For this review, take the finished solid that the model builds, in its own axes (mm). A direction names the side the tool comes from. Give positions to 0.01 mm unless a question says otherwise; leave off trailing zeros. Loops run counter-clockwise (first coordinate to the right, second up) from the corner with the lowest first, then second, coordinate; pieces in that order, holes last. Notation, with made-up numbers: (-8.5, 49.5) -> (31.5, 49.5) arc R16 ccw to (31.5, 55.5) -> close; hole circle Ø4 at (-16.5, 55). An arc over 180 degrees is marked (long way). One line per question, with ' | ' between items. Start each with the question number.
(1) Draft analysis for pull direction X (two halves, no side actions). For faces 1 (the flat face through (-20.3, 2, 0)), 2 (the cylindrical face through (20.72, -20.49, 24.65)), 3 (the cylindrical face through (-17.15, 16.99, 24.65)), state which applies: +X half, -X half, draft (parallel to the pull), parting line (faces both ways), or undercut.
(2) Consider section B-B (y = 375). Write out the cut boundary in (x, z), and give its area (3 significant figures).
(3) Consider section A-A (x = 0). Write out the cut boundary in (y, z), and give its area (3 significant figures).
(4) Insertion check: P1, Ø5, axis at x = 14, z = 31.5, coming from the +Y side; P2, Ø16, axis at x = -4, z = 30.5, coming from the +Y side; P3, Ø5, axis at x = 14.5, y = 231, coming from the +Z side. Each pin has a flat end and moves straight along its axis. Give the tip position at first contact, or say it passes through.
(5) Tool access review of faces 4 (the flat face through (-20.3, 2, 50)), 5 (the flat face through (0, -25, 25)), 6 (the cylindrical face through (-16.99, -17.15, 24.65)): name each direction out of +Z, -Z, +X, -X, +Y, -Y from which nothing blocks a thin tool from reaching the whole face with its end or side.
(6) Consider section C-C (z = 64.5). Write out the cut boundary in (x, y), and give its area (3 significant figures).
(7) Consider section D-D (y = 296). Write out the cut boundary in (x, z), and give its area (3 significant figures).
(8) Wall thickness on probe 1 along Y at (x, z) = (0, 14); probe 2 along Y at (x, z) = (2, 34); probe 3 along Z at (x, y) = (0, 319): over which ranges is each line inside the solid? List them lowest first.
from build123d import *

# Parameters (mm, degrees)
EXTRUDE_1_DEPTH     = 50
SKETCH_2_W          = 40
SKETCH_2_H          = 40
EXTRUDE_2_DEPTH     = 600
FILLET_1_RADIUS     = 20
FILLET_1_LENGTH     = 40
SKETCH_5_R          = 7.5
EXTRUDE_4_DEPTH     = 30
SKETCH_6_R          = 15
CUT_EXTRUDE_1_DEPTH = 631.892225344


with BuildPart() as part:
    # 草图1 → 凸台-拉伸1 (new body)
    with BuildSketch(Plane.XY):
        with BuildLine():
            Line((-10, 25), (10, 25))
            ThreePointArc((10, 25), (20.606601718, 20.606601718), (25, 10))
            Line((25, 10), (25, -10))
            ThreePointArc((25, -10), (20.606601718, -20.606601718), (10, -25))
            Line((10, -25), (-10, -25))
            ThreePointArc((-10, -25), (-20.606601718, -20.606601718), (-25, -10))
            Line((-25, -10), (-25, 10))
            ThreePointArc((-25, 10), (-20.606601718, 20.606601718), (-10, 25))
        make_face()
        with BuildLine():
            Line((-10, 20), (10, 20))
            ThreePointArc((10, 20), (17.071067812, 17.071067812), (20, 10))
            Line((20, 10), (20, -10))
            ThreePointArc((20, -10), (17.071067812, -17.071067812), (10, -20))
            Line((10, -20), (-10, -20))
            ThreePointArc((-10, -20), (-17.071067812, -17.071067812), (-20, -10))
            Line((-20, -10), (-20, 10))
            ThreePointArc((-20, 10), (-17.071067812, 17.071067812), (-10, 20))
        make_face(mode=Mode.SUBTRACT)
    extrude(amount=EXTRUDE_1_DEPTH)

    # 草图2 → 凸台-拉伸2 (add)
    with BuildSketch(Plane(origin=(0, 25, 0), x_dir=(1, 0, 0), z_dir=(0, 1, 0))):
        with Locations((0, -25)):
            Rectangle(SKETCH_2_W, SKETCH_2_H)
    extrude(amount=EXTRUDE_2_DEPTH)

    # 圆角1: full round fillet: the end face becomes a half cylinder, R = half its width
    fillet_1_face = Plane((0, 625, 25), x_dir=(0, 0, -1), z_dir=(0, 1, 0))  # on the end face: x along it, z out of the body
    fillet_1_slab = fillet_1_face.offset(-FILLET_1_RADIUS / 2) * Box(FILLET_1_LENGTH, 2 * FILLET_1_RADIUS, FILLET_1_RADIUS, mode=Mode.PRIVATE)  # the body's end, R deep
    fillet_1_round = Plane((0, 605, 25), x_dir=(0, 1, 0), z_dir=(0, 0, -1)) * Cylinder(FILLET_1_RADIUS, FILLET_1_LENGTH, mode=Mode.PRIVATE)  # its axis R under the face
    add(fillet_1_slab - fillet_1_round, mode=Mode.SUBTRACT)

    # 草图5 → 凸台-拉伸4 (add)
    with BuildSketch(Plane.XY.offset(45)):
        with Locations(Location((0, 605, 0), (0, 0, 180))):
            Circle(SKETCH_5_R)
    extrude_4 = extrude(amount=EXTRUDE_4_DEPTH)

    # 镜向2: 凸台-拉伸4 across plane
    add(extrude_4.mirror(Plane.XY.offset(25)))

    # 草图6 → 切除-拉伸1 (cut, through all)
    with BuildSketch(Plane(origin=(25, 0, 45), x_dir=(1, 0, 0), z_dir=(0, 0, 1))):
        with Locations((-25, 375)):
            Circle(SKETCH_6_R)
    extrude(amount=-CUT_EXTRUDE_1_DEPTH, mode=Mode.SUBTRACT)


solid = part.part
A:
1) face 1: draft | face 2: +X half | face 3: undercut
2) outline: (-20, 5) -> (-15, 5) -> (-15, 45) -> (-20, 45) -> close; (15, 5) -> (20, 5) -> (20, 45) -> (15, 45) -> close | area: 400 mm^2
3) outline: (-25, 0) -> (-20, 0) -> (-20, 50) -> (-25, 50) -> close; (20, 0) -> (25, 0) -> (25, 5) -> (360, 5) -> (360, 45) -> (25, 45) -> (25, 50) -> (20, 50) -> close; (390, 5) -> (597.5, 5) -> (597.5, -25) -> (612.5, -25) -> (612.5, 5) -> (625, 5) -> (625, 45) -> (612.5, 45) -> (612.5, 75) -> (597.5, 75) -> (597.5, 45) -> (390, 45) -> close | area: 24,200 mm^2
4) P1: stops at y = 621.36 | P2: stops at y = 625 | P3: stops at z = 45
5) face 4: +Z, +X, -X, -Y | face 5: +Z, -Z, +X, -X, -Y | face 6: +Z, -Z
6) outline: circle Ø15 at (0, 605) | area: 177 mm^2
7) outline: (-20, 5) -> (20, 5) -> (20, 45) -> (-20, 45) -> close | area: 1,600 mm^2
8) probe 1: y = -25 to -20, 20 to 360, 390 to 625 | probe 2: y = -25 to -20, 20 to 360.13, 389.87 to 624.9 | probe 3: z = 5 to 45
